Autodesk Inventor part; units mm, degrees
ref_plane "YZ Plane" through (0, 0, 0) normal (1, 0, 0) x (0, 1, 0)
ref_plane "XZ Plane" through (0, 0, 0) normal (0, 1, 0) x (-1, 0, 0)
ref_plane "XY Plane" through (0, 0, 0) normal (0, 0, 1) x (1, 0, 0)
sketch "Sketch1" plane through (0, 0, 0) normal (0, 1, 0) x (-1, 0, 0)
  arc A0 (-48.1285, 3.1733) -> (48.1285, 3.1733) centre (0, 0) ccw
  arc A1 (-45.058, 0) -> (45.058, 0) centre (0, 0) ccw
  arc A2 (-38.708, 0) -> (38.708, 0) centre (0, 0) ccw
  arc A3 (-51.408, 0) -> (51.408, 0) centre (0, 0) ccw
  arc A4 (-57.758, 0) -> (57.758, 0) centre (0, 0) ccw
  circle A5 centre (48.233, 0) radius 3.175
  line L0 (0, 0) -> (48.233, 0)
  line L1 (0, 0) -> (-48.233, 0)
  circle A6 centre (-48.233, 0) radius 3.175
  line L2 (-48.233, 0) -> (-48.233, 15.24)
  line L3 (-38.708, 0) -> (-38.708, 15.24)
  line L4 (-57.758, 0) -> (-57.758, 15.24)
  line L5 (48.233, 0) -> (48.233, 15.24)
  line L6 (38.708, 0) -> (38.708, 15.24)
  line L7 (57.758, 0) -> (57.758, 15.24)
  line L8 (-38.708, 21.59) -> (-57.758, 21.59)
  line L9 (-57.758, 21.59) -> (-57.758, 15.24)
  line L10 (-38.708, 21.59) -> (-38.708, 15.24)
  line L11 (57.758, 21.59) -> (38.708, 21.59)
  line L12 (38.708, 21.59) -> (38.708, 15.24)
  line L13 (57.758, 21.59) -> (57.758, 15.24)
  point P0 (-48.233, 15.24)
  point P1 (45.058, 0)
  dimension "d0" = 96.4661
  dimension "d1" = 3.175
  dimension "d2" = 6.35
  dimension "d3" = 3.175
  dimension "d4" = 6.35
  dimension "d5" = 6.35
  dimension "d6" = 6.35
  dimension "d7" = 15.24
  dimension "d8" = 15.24
  dimension "d18" = 6.35
  dimension "d19" = 6.35
extrude "Extrusion1" add sketch "Sketch1" along normal blind 3.175 contours A6 A3 A5 L0 L6 L12 L11 L13 L7 A4 L4 L9 L8 L10 L3 L1 | L1 A2 L0 A1
hole "Hole1" at (48.233, 0, 15.24) at (-48.233, 0, 15.24) direction (0, 1, 0) diameter 4.9784 end through all
equation "\"d0\" = ringDiam"
equation "\"d7\" = thickness + stageSpace"
equation "\"d8\" = thickness + stageSpace"
equation "\"height\" = 203.2"
equation "\"thickness\" = 12.7"
equation "\"shaftDiam\" = 6.35"
equation "\"shaftSpace\" = 1.5875"
equation "\"stageSpace\" = 2.54"
equation "\"stageAngle\" = 15deg"
equation "\"bearingDiam\" = 9.5504"
equation "\"FlangeDiam\" = 12.7"
equation "\"FlangeDepth\" = 1.5875"
equation "\"smallFilet\" = 0.39687"
equation "\"ringDiam\" = 96.46608"
equation "\"stockHeight\" = 50.8"
equation "\"stockWidth\" = 76.2"
equation "\"stockRad\" = 9.525"
equation "\"stockGuage\" = 3.175"
equation "\"groundActu\" = 304.8"
equation "\"baseWidth\" = 1066.8"
equation "\"baseDepth\" = 254"
equation "\"capThickness\" = 3.175"
equation "\"sup1Len\" = 660.4"
equation "\"sup1Ang\" = 22.619865deg"
equation "\"sup2Len\" = 2079.37366"
equation "\"sup2Ang\" = 8.959949deg"
equation "\"supVertLen\" = 955.13561"
equation "\"supSideLen\" = 1531.12879"
equation "\"supSideAng\" = 19.376933deg"
properties part number "lock ring 1" material "Aluminum 6061"
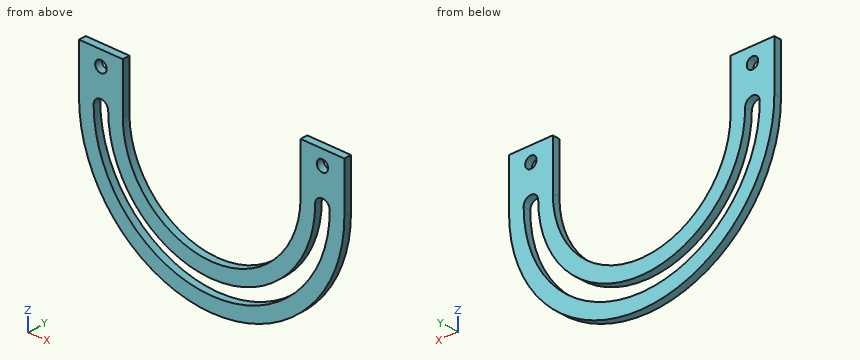
CAD build for the part. Positions are in the model's coordinates, mm. Give positions to 0.01 mm unless a question says otherwise; leave off trailing zeros. Loops run counter-clockwise (first coordinate to the right, second up) from the corner with the lowest first, then second, coordinate; pieces in that order, holes last. Notation, with made-up numbers: (75, 83.25) - (122, 83.25) arc R34 cw to (122, 116.25) - close; hole circle Ø11 at (80.5, 49.25). An arc over 180 degrees is marked (long way). Put each result on its own line as item: value.
Q1. Slice it at A-A (z = 4.5). Give the cut face in (x, y) (3 decimals), plus the area to 3 significant figures.
Filled in:
outline: (-57.758, 0) - (-38.708, 0) - (-38.708, 3.175) - (-57.758, 3.175) - close; (38.708, 0) - (57.758, 0) - (57.758, 3.175) - (38.708, 3.175) - close
area: 121 mm²
Q2. Slice it at D-D (z = -40). Give the cut face in (x, y) (3 decimals).
Filled in:
outline: (-41.665, 0) - (-32.292, 0) - (-32.292, 3.175) - (-41.665, 3.175) - close; (-20.742, 0) - (20.742, 0) - (20.742, 3.175) - (-20.742, 3.175) - close; (32.292, 0) - (41.665, 0) - (41.665, 3.175) - (32.292, 3.175) - close
Q3. Slice it at C-C (z = 15.24). Give the cut face in (x, y) (3 decimals), plus the area to 3 significant figures.
Filled in:
outline: (-57.758, 0) - (-50.722, 0) - (-50.722, 3.175) - (-57.758, 3.175) - close; (-45.744, 0) - (-38.708, 0) - (-38.708, 3.175) - (-45.744, 3.175) - close; (38.708, 0) - (45.744, 0) - (45.744, 3.175) - (38.708, 3.175) - close; (50.722, 0) - (57.758, 0) - (57.758, 3.175) - (50.722, 3.175) - close
area: 89.4 mm²
Q4. Probe line 1 along X through (y, z) = (1.3, 15.24); line 2 along X through (y, z) = (2, -40.5); line 3 along X through (y, z) = (0.35, -30). List the from-to ranges inside material, lowest first.
Filled in:
line 1: x = -57.76 to -50.72, -45.74 to -38.71, 38.71 to 45.74, 50.72 to 57.76
line 2: x = -41.18 to -31.66, -19.75 to 19.75, 31.66 to 41.18
line 3: x = -49.36 to -41.75, -33.62 to -24.46, 24.46 to 33.62, 41.75 to 49.36
Q5. Slice it at B-B (x = 0). Give the cut face in (y, z) (3 decimals).
Filled in:
outline: (0, -57.758) - (3.175, -57.758) - (3.175, -51.408) - (0, -51.408) - close; (0, -45.058) - (3.175, -45.058) - (3.175, -38.708) - (0, -38.708) - close
Q6. Flat gauge pins, fed straight in: pin 1 (1.5 mm diameter, centred on x = 16.5, y = 1.5, fed in from +Z); pin 2 (1.5 mm diameter, centred on x = 13.5, y = 2, fed in from +Z). Where does each tip first touch, or does it go through?
Filled in:
pin 1: stops at z = -34.65
pin 2: stops at z = -35.99
